Autodesk Inventor part; units mm, degrees
ref_plane "YZ Plane" through (0, 0, 0) normal (1, 0, 0) x (0, 1, 0)
ref_plane "XZ Plane" through (0, 0, 0) normal (0, 1, 0) x (-1, 0, 0)
ref_plane "XY Plane" through (0, 0, 0) normal (0, 0, 1) x (1, 0, 0)
sketch "草圖1" plane through (0, 0, 0) normal (0, 1, 0) x (-1, 0, 0)
  line L0 (0, 0) -> (-40, 0)
  line L1 (-40, 0) -> (-40, -40)
  line L2 (-40, -40) -> (0, -40)
  line L3 (0, -40) -> (0, 0)
  dimension "d0" = 40
  dimension "d1" = 40
extrude "擠出1" add sketch "草圖1" along normal blind 10
sketch "草圖2" plane through (40, 0, -40) normal (0, 0, -1) x (-1, 0, 0)
  line L0 (40, 0) -> (0, 0)
  line L1 (40, 0) -> (-30, 0)
  line L2 (-30, 0) -> (-30, 50)
  line L3 (-30, 50) -> (40, 50)
  line L4 (40, 50) -> (40, 0)
  line L5 (40, 10) -> (0, 10)
  line L6 (40, 10) -> (60, 10)
  line L7 (60, 10) -> (60, 50)
  line L8 (60, 50) -> (40, 50)
  line L9 (40, 50) -> (40, 10)
  line L10 (0, 0) -> (0, 10)
  dimension "d4" = 40
  dimension "d5" = 30
  dimension "d6" = 20
extrude "擠出2" add sketch "草圖2" along normal blind 10
fillet "圓角1" radius 20 2 edges at (-20, 50, -45) (-20, 10, -45)
chamfer "倒角1" distance 40 angle 45 1 edges at (70, 50, -45)
fillet "圓角2" radius 20 2 edges at (0, 5, 0) (40, 5, 0)
hole "孔1" at (20, 10, -20) direction (0, -1, 0) diameter 20 depth 10 tip angle 118
hole "孔2" at (0, 30, -40) direction (0, 0, -1) diameter 20 depth 20 tip angle 118
properties part number "25"
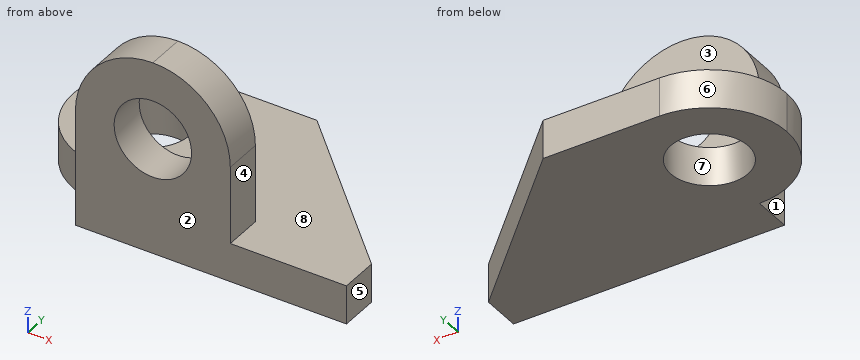
Geometry check sheet. Reference: the model listing, model coordinates, mm. Face numbers are marked on the shaded views. A direction names the side the tool comes from. Coordinates: 2 decimals unless noted, no trailing zeros. Order: outer loops, then holes, each group sorted by start corner. A loop starts at its lowest first (then second) coordinate and runs counter-clockwise, first axis right, second up. Notation, with made-up numbers: (-21, 50.5) - (34, 50.5) arc R29 cw to (34, 83.5) - close; hole circle Ø6 at (57.5, 16). An arc over 180 degrees is marked (long way). One line per item, written item: value.
(1) Thickness scan on probe 1 along X at (y, z) = (6.5, -20); probe 2 along X at (y, z) = (30, -44); probe 3 along Z at (x, y) = (34, 39). Record the ranges inside material, lowest first. Write a range as from..to.
Data:
probe 1: x = 0..10, 30..40
probe 2: x = -20..-10, 10..50
probe 3: z = -50..-40
(2) Sectioned sample at A-A (y = 28). Enter the section's corners in (x, z), and give its area (3 significant figures).
Data:
outline: (-19.9, -50) - (-9.8, -50) - (-9.8, -40) - (-19.9, -40) - close; (9.8, -50) - (52, -50) - (52, -40) - (9.8, -40) - close
area: 523 mm^2
(3) Access from +Z, -Z, +X, -X, +Y, -Y to the whole of each face (thin tool, end or side, straight path). Record for the marked faces 1, 2, 3, 4 and 5.
Data:
face 1: +Z, -Z, -X, -Y
face 2: +Z, -Z, +X, -X, -Y
face 3: +Z, +X, -X, +Y
face 4: +Z, +X, +Y, -Y
face 5: +Z, -Z, +X, +Y, -Y
(4) Sectioned sample at C-C (x = 55.5). Enter the section's corners in (y, z).
Data:
outline: (0, -50) - (24.5, -50) - (24.5, -40) - (0, -40) - close
(5) Release check for a two-part mould opening along Y. For the marked faces 6, 7 and 8 record: +Y half, -Y half, draft (parallel to the pull), parting line (faces both ways), or undercut.
Data:
face 6: +Y half
face 7: undercut
face 8: draft
(6) Depth check by flat-ended pin: pin 1 Ø4 at (x, y) = (50.5, 12.5) entering from +Z; pin 2 Ø16 at (x, y) = (0, 30) entering from +Z; pin 3 Ø3 at (y, z) = (2.5, -28) entering from +X; pin 4 Ø11 at (y, z) = (3.5, -29) entering from -X. Enter the tip coordinate at first touch or a pass-through.
Data:
pin 1: stops at z = -40
pin 2: passes through
pin 3: stops at x = 40
pin 4: stops at x = 0
(7) Sectioned sample at B-B (z = -18). Enter the section's corners in (x, y), and give its area (3 significant figures).
Data:
outline: (0.1, 0) - (10.2, 0) - (10.2, 10) - (0.1, 10) - close; (29.8, 0) - (39.9, 0) - (39.9, 10) - (29.8, 10) - close
area: 202 mm^2
(8) Sectioned sample at D-D (y = 42). Enter the section's corners in (x, z), and give its area (3 significant figures).
Data:
outline: (-16, -50) - (38, -50) - (38, -40) - (-16, -40) - close
area: 540 mm^2
